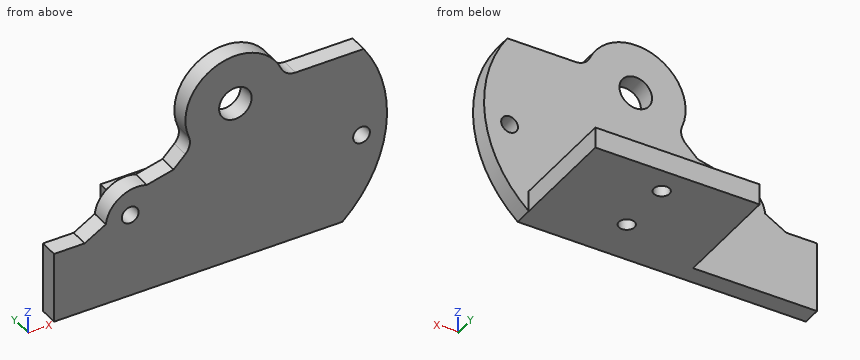
```python
from build123d import *
from build123d.topology import SkipClean

# Parameters (mm, degrees)
CROQUIS1_W              = 70
CROQUIS1_H              = 65
EXTRUIR1_DEPTH          = 3.5
CROQUIS2_R              = 3.1
EXTRUIR2_DEPTH          = 5
EXTRUIR3_DEPTH          = 10
CROQUIS4_OUTSIDE_W      = 91.294
CROQUIS4_OUTSIDE_H      = 86.294
EXTRUIR4_DEPTH          = 10
REDONDEO1_R             = 3
EXTRUIR5_DEPTH          = 13.5
EXTRUIR6_DEPTH          = 3.5
CROQUIS7_R              = 1.6
EXTRUIR7_DEPTH          = 47.982330447
CROQUIS8_R              = 3.1
EXTRUIR8_DEPTH          = 5
CROQUIS9_W              = 0.7
CROQUIS9_H              = 10.5
EXTRUIR9_DEPTH          = 10
EXTRUIR10_DEPTH         = 63.752948337
EXTRUIR10_DEPTH_BACK    = 10
CROQUIS10_W             = 3.0625
CROQUIS10_H             = 5
CROQUIS11_W             = 54.8364
CROQUIS11_H             = 21.05596306
SALIENTE_EXTRUIR1_DEPTH = 4
CROQUIS15_W             = 23.581168674
CROQUIS15_H             = 21.05596306
CORTAR_EXTRUIR3_DEPTH   = 10
CROQUIS16_R             = 1.5
CORTAR_EXTRUIR4_DEPTH   = 10


with BuildPart() as part:
    # Croquis1 → Extruir1 (new body)
    with BuildSketch(Plane(origin=(0, 0, 0), x_dir=(1, 0, 0), z_dir=(0, 1, 0))):
        Rectangle(CROQUIS1_W, CROQUIS1_H)
    extrude(amount=EXTRUIR1_DEPTH)

    # Croquis2 → Extruir2 (cut)
    with BuildSketch(Plane(origin=(0, 3.5, 0), x_dir=(1, 0, 0), z_dir=(0, 1, 0))):
        with Locations(Location((0, -17.5, 0), (0, 0, 270))):
            Circle(CROQUIS2_R)
    extrude(amount=-EXTRUIR2_DEPTH, mode=Mode.SUBTRACT)

    # Croquis3 → Extruir3 (add)
    with BuildSketch(Plane(origin=(0, 3.5, 0), x_dir=(1, 0, 0), z_dir=(0, 1, 0))):
        with BuildLine():
            Line((-34.4868, 13.5), (20.3496, 13.5))
            Line((20.3496, 13.5), (20.3496, 0))
            Line((20.3496, 0), (17.146428199, 0))
            ThreePointArc((17.146428199, 0), (22.955777517, -8.939493087), (24.418230894, -19.5))
            Line((24.418230894, -19.5), (9.287087811, -19.5))
            ThreePointArc((9.287087811, -19.5), (-3.635492607, -26.276855559), (-7.981176331, -12.347250794))
            Line((-7.981176331, -12.347250794), (-18.680510212, -1.647916913))
            ThreePointArc((-18.680510212, -1.647916913), (-17.932408832, -0.806327142), (-17.146428199, 0))
            Line((-17.146428199, 0), (-34.4868, 0))
            Line((-34.4868, 0), (-34.4868, 13.5))
        make_face()
        with BuildLine():
            Line((-32.9868, 1.5), (-12.961481397, 1.5))
            ThreePointArc((-12.961481397, 1.5), (-14.868021343, 0.048274597), (-16.613165932, -1.593940849))
            Line((-16.613165932, -1.593940849), (-5.999348286, -12.207758495))
            ThreePointArc((-5.999348286, -12.207758495), (-3.061467459, -24.89103626), (7.984359711, -18))
            Line((7.984359711, -18), (22.994564575, -18))
            ThreePointArc((22.994564575, -18), (20.451694563, -6.977253708), (12.961481397, 1.5))
            Line((12.961481397, 1.5), (18.8496, 1.5))
            Line((18.8496, 1.5), (18.8496, 12))
            Line((18.8496, 12), (-32.9868, 12))
            Line((-32.9868, 12), (-32.9868, 1.5))
        make_face(mode=Mode.SUBTRACT)
    extrude(amount=EXTRUIR3_DEPTH)

    # Croquis4 outside → Extruir4 (cut)
    with SkipClean():  # the faces are left unmerged after this step: merging them gives an invalid solid
        with BuildSketch(Plane(origin=(0, 3.5, 0), x_dir=(1, 0, 0), z_dir=(0, 1, 0))):
            Rectangle(CROQUIS4_OUTSIDE_W, CROQUIS4_OUTSIDE_H)
            with BuildLine():
                Line((-34.4868, 0), (-17.146428199, 0))
                ThreePointArc((-17.146428199, 0), (-17.932408832, -0.806327142), (-18.680510212, -1.647916913))
                Line((-18.680510212, -1.647916913), (-7.981176331, -12.347250794))
                ThreePointArc((-7.981176331, -12.347250794), (-3.635492607, -26.276855559), (9.287087811, -19.5))
                Line((9.287087811, -19.5), (24.418230894, -19.5))
                ThreePointArc((24.418230894, -19.5), (22.955777517, -8.939493087), (17.146428199, 0))
                Line((17.146428199, 0), (20.3496, 0))
                Line((20.3496, 0), (20.3496, 13.5))
                Line((20.3496, 13.5), (-34.4868, 13.5))
                Line((-34.4868, 13.5), (-34.4868, 0))
            make_face(mode=Mode.SUBTRACT)
        extrude(amount=-EXTRUIR4_DEPTH, mode=Mode.SUBTRACT)

    # Redondeo1
    redondeo1_edges = [part.edges().sort_by_distance(p)[0] for p in [
        (-7.981176331, 8.5, 12.347250794),
        (9.287087811, 8.5, 19.5),
        (-5.999348286, 8.5, 12.207758495),
        (7.984359711, 8.5, 18),
    ]]
    fillet(redondeo1_edges, radius=REDONDEO1_R)

    # Croquis5 → Extruir5 (add)
    with SkipClean():  # the faces are left unmerged after this step: merging them gives an invalid solid
        with BuildSketch(Plane.XZ):
            with BuildLine():
                Line((-18.680510212, 1.647916913), (-14.437869525, 5.8905576))
                ThreePointArc((-14.437869525, 5.8905576), (-21.723092903, 6.819250451), (-24.449770984, 0))
                Line((-24.449770984, 0), (-17.146428199, 0))
                ThreePointArc((-17.146428199, 0), (-17.932408832, 0.806327142), (-18.680510212, 1.647916913))
            make_face()
            with BuildLine():
                Line((20.3496, 0), (20.3496, -13.5))
                ThreePointArc((20.3496, -13.5), (28.665212431, 2.225567304), (24.418230894, 19.5))
                ThreePointArc((24.418230894, 19.5), (22.955777517, 8.939493087), (17.146428199, 0))
                Line((17.146428199, 0), (20.3496, 0))
            make_face()
        extrude(amount=-EXTRUIR5_DEPTH)

    # Chaflán1
    # the kernel refuses this chamfer: 5, 4.044665138 mm, written as the material it adds along each edge
    with BuildSketch(Plane(origin=(-14.437869525, 3.5, 5.8905576), x_dir=(-0.8768595348589333, 0, 0.4807466652270976), z_dir=(0, 1, 0))) as chafl_n1_piece_1:
        with BuildLine():
            Line((2.949791971, 0), (-1.211824758, 3.780414953))
            Line((-1.211824758, 3.780414953), (-1.307822013, 3.752405544))
            ThreePointArc((-1.307822013, 3.752405544), (-0.651776703, 1.876825504), (-0.095997255, -0.02800941))
            Line((-0.095997255, -0.02800941), (0.02800941, -0.095997255))
            ThreePointArc((0.02800941, -0.095997255), (1.47002525, 0.136406993), (2.931105495, -0.098238565))
            Line((2.931105495, -0.098238565), (2.949791971, 0))
        make_face()
    extrude(amount=10)
    with BuildSketch(Plane(origin=(-24.449770984, 3.5, 0), x_dir=(-0.008036803743584595, 0, 0.9999677043712897), z_dir=(0, 1, 0))) as chafl_n1_piece_2:
        with BuildLine():
            Line((2.423263449, 0), (-0.064845869, -4.38542071))
            Line((-0.064845869, -4.38542071), (-0.164842639, -4.386224391))
            ThreePointArc((-0.164842639, -4.386224391), (-0.082377051, -2.193111839), (-0.09999677, -0.00080368))
            Line((-0.09999677, -0.00080368), (0.026691621, 0.096371974))
            ThreePointArc((0.026691621, 0.096371974), (1.204598314, -0.104316531), (2.411212242, 0.099271186))
            Line((2.411212242, 0.099271186), (2.423263449, 0))
        make_face()
    extrude(amount=10)
    with BuildSketch(Plane(origin=(-24.449770984, 0, 0), x_dir=(-0.9997395779240649, 0, -0.022820524363231526), z_dir=(0, 1, 0))) as chafl_n1_piece_3:
        with BuildLine():
            Line((4.385900112, 0), (-0.035828136, 2.422998574))
            Line((-0.035828136, 2.422998574), (-0.134910293, 2.409480951))
            ThreePointArc((-0.134910293, 2.409480951), (0.08649505, 1.206008973), (-0.096756078, 0.025263837))
            Line((-0.096756078, 0.025263837), (0.002282052, -0.099973958))
            ThreePointArc((0.002282052, -0.099973958), (2.194090072, -0.04994272), (4.388182164, -0.099973958))
            Line((4.388182164, -0.099973958), (4.385900112, 0))
        make_face()
    extrude(amount=3.5)
    with BuildSketch(Plane(origin=(-14.437869525, 0, 5.8905576), x_dir=(0.7254657554746632, 0, 0.6882582637597433), z_dir=(0, 1, 0))) as chafl_n1_piece_4:
        with BuildLine():
            Line((3.96989376, 0), (-0.900434913, -2.809001538))
            Line((-0.900434913, -2.809001538), (-0.98828054, -2.761219262))
            ThreePointArc((-0.98828054, -2.761219262), (-0.318834214, -1.441501248), (-0.099965384, 0.002630967))
            Line((-0.099965384, 0.002630967), (0.002630967, 0.099965384))
            ThreePointArc((0.002630967, 0.099965384), (1.986203869, 0.047760165), (3.972524727, 0.099965384))
            Line((3.972524727, 0.099965384), (3.96989376, 0))
        make_face()
    extrude(amount=3.5)


with BuildPart() as body_2:
    # Croquis6 → Extruir6 (new body)
    with BuildSketch(Plane(origin=(0, 13.5, 0), x_dir=(1, 0, 0), z_dir=(0, 1, 0))):
        with BuildLine():
            Line((-34.4868, 13.5), (-34.4868, 0))
            Line((-34.4868, 0), (-28.661374979, 0))
            Line((-28.661374979, 0), (-24.642400208, -2.323096648))
            ThreePointArc((-24.642400208, -2.323096648), (-21.929637735, -6.692039268), (-16.829963308, -7.355409896))
            Line((-16.829963308, -7.355409896), (-11.752306982, -8.576120143))
            Line((-11.752306982, -8.576120143), (-9.515139435, -10.813287689))
            ThreePointArc((-9.515139435, -10.813287689), (-8.69974084, -12.321679102), (-8.843709432, -14.030302105))
            ThreePointArc((-8.843709432, -14.030302105), (-3.635492607, -26.276855559), (8.70689382, -21.3))
            ThreePointArc((8.70689382, -21.3), (9.813271565, -19.99001992), (11.456439237, -19.5))
            Line((11.456439237, -19.5), (24.418230894, -19.5))
            ThreePointArc((24.418230894, -19.5), (28.665212431, -2.225567304), (20.3496, 13.5))
            Line((20.3496, 13.5), (-34.4868, 13.5))
        make_face()
    extrude(amount=EXTRUIR6_DEPTH)


with BuildPart() as extruir7_tool:
    # Croquis7 → Extruir7 (new, through all)
    with BuildSketch(Plane(origin=(0, 17, 0), x_dir=(1, 0, 0), z_dir=(0, 1, 0))):
        with Locations(Location((-20, -2.5, 0), (0, 0, 270))):
            Circle(CROQUIS7_R)
        with Locations(Location((24, -2.5, 0), (0, 0, 270))):
            Circle(CROQUIS7_R)
    extrude(amount=-EXTRUIR7_DEPTH)


with BuildPart() as part_1:
    add(part.part)

    # Extruir7: cut by extruir7_tool
    add(extruir7_tool.part, mode=Mode.SUBTRACT)

    # Croquis9 → Extruir9 (cut)
    with BuildSketch(Plane(origin=(0, 13.5, 0), x_dir=(1, 0, 0), z_dir=(0, 1, 0))):
        with Locations((19.1996, 6.75)):
            Rectangle(CROQUIS9_W, CROQUIS9_H)
    extrude(amount=-EXTRUIR9_DEPTH, mode=Mode.SUBTRACT)

    # Croquis10 → Extruir10 (cut, two sides: drawn at the far end of the back side and taken through both)
    with BuildSketch(Plane.ZY.offset(-19.5496).offset(-EXTRUIR10_DEPTH_BACK)):
        with Locations((-8.9375, 8.5)):
            Rectangle(CROQUIS10_W, CROQUIS10_H)
    extrude(amount=EXTRUIR10_DEPTH + EXTRUIR10_DEPTH_BACK, mode=Mode.SUBTRACT)


with BuildPart() as body_2_1:
    add(body_2.part)

    # Extruir7: cut by extruir7_tool
    add(extruir7_tool.part, mode=Mode.SUBTRACT)

    # Croquis8 → Extruir8 (cut)
    with BuildSketch(Plane(origin=(0, 17, 0), x_dir=(1, 0, 0), z_dir=(0, 1, 0))):
        with Locations(Location((0, -17.5, 0), (0, 0, 270))):
            Circle(CROQUIS8_R)
    extrude(amount=-EXTRUIR8_DEPTH, mode=Mode.SUBTRACT)

    # Croquis11 → Saliente-Extruir1 (add)
    with BuildSketch(Plane(origin=(0, 0, -13.5), x_dir=(-1, 0, 0), z_dir=(0, 0, -1))):
        with Locations((7.0686, 27.52798153)):
            Rectangle(CROQUIS11_W, CROQUIS11_H)
    extrude(amount=-SALIENTE_EXTRUIR1_DEPTH)

    # Croquis15 → Cortar-Extruir3 (cut)
    with BuildSketch(Plane.XY.offset(-9.5)):
        with Locations((-22.696215663, 27.52798153)):
            Rectangle(CROQUIS15_W, CROQUIS15_H)
    extrude(amount=-CORTAR_EXTRUIR3_DEPTH, mode=Mode.SUBTRACT)

    # Croquis16 → Cortar-Extruir4 (cut)
    with BuildSketch(Plane.XY.offset(-9.5)):
        with Locations((4.721984337, 33.05596306)):
            Circle(CROQUIS16_R)
        with Locations((4.721984337, 22)):
            Circle(CROQUIS16_R)
    extrude(amount=-CORTAR_EXTRUIR4_DEPTH, mode=Mode.SUBTRACT)


solid = body_2_1.part
```
Can you work these out from the model? Positions are in its coordinate system, mm. Give positions to 0.01 mm unless a question says otherwise; leave off trailing zeros. Loops run counter-clockwise (first coordinate to the right, second up) from the corner with the lowest first, then second, coordinate; pieces in that order, holes last. Notation, with made-up numbers: M 21.5,57.25 L 65.5,57.25 A22 cw 65.5,68.25 Z; hole C -4.75,6 d2. An arc over 180 degrees is marked long. One line per question, with ' | ' between items. Start each with the question number.
Q1. If we section it at A-A (x = 0): Please give me the cut outline in (y, z).
Q2. If we section it at C-C (z = 17.5): Please give me the cut outline in (x, y), plus the area to 3 significant figures.
Q3. If we section it at B-B (y = 22): Please give me the cut outline in (x, z).
Q4. For pin 1 Ø6 at (y, z) = (17.5, 13.5) entering from +X; pin 2 Ø1 at (x, y) = (-31.5, 15) entering from +Z; pin 3 Ø10 at (x, z) = (0, 17.5) entering from +Y, each with a flat end and sliding along its axis, tell me the tip position at first contact or that it passes through.
Q5. If we section it at D-D (y = 36): Please give me the cut outline in (x, z), plus the area to 3 significant figures.
Q6. If I drill on line 1 (Y direction, x = 9.5, z = -8.5); line 2 (Z direction, x = -3, y = 29); line 3 (Z direction, x = -23, y = 14.75), over which ranges is the centre line in solid material (lowest first)? Write a range as from..to.
Computed:
1) outline: M 13.5,-13.5 L 38.06,-13.5 L 38.06,-9.5 L 17,-9.5 L 17,14.4 L 13.5,14.4 Z; M 13.5,20.6 L 17,20.6 L 17,27 L 13.5,27 Z
2) outline: M -9.5,13.5 L -3.1,13.5 L -3.1,17 L -9.5,17 Z; M 3.1,13.5 L 25.67,13.5 L 25.67,17 L 3.1,17 Z | area: 101 mm²
3) outline: M -10.91,-13.5 L 3.22,-13.5 L 3.22,-9.5 L -10.91,-9.5 Z; M 6.22,-13.5 L 20.35,-13.5 L 20.35,-9.5 L 6.22,-9.5 Z
4) pin 1: stops at x = 28.29 | pin 2: stops at z = 0 | pin 3: stops at y = 17
5) outline: M -10.91,-13.5 L 20.35,-13.5 L 20.35,-9.5 L -10.91,-9.5 Z | area: 125 mm²
6) line 1: y = 13.5..17 | line 2: z = -13.5..-9.5 | line 3: z = -13.5..5.81
